Autodesk Inventor part; units mm, degrees
ref_plane "YZ Plane" through (0, 0, 0) normal (1, 0, 0) x (0, 1, 0)
ref_plane "XZ Plane" through (0, 0, 0) normal (0, 1, 0) x (-1, 0, 0)
ref_plane "XY Plane" through (0, 0, 0) normal (0, 0, 1) x (1, 0, 0)
sketch "Sketch1" plane through (0, 0, 0) normal (0, 1, 0) x (-1, 0, 0)
  circle A0 centre (0, 0) radius 12.3
  circle A1 centre (0, 0) radius 4.5
  circle A2 centre (0, 0) radius 2.75
  circle A3 centre (0, 0) radius 1.5
  dimension "d0" = 24.6
  dimension "d1" = 9
  dimension "d2" = 5.5
  dimension "d3" = 3
extrude "Extrusion1" add sketch "Sketch1" along normal blind 2 contours A0
sketch "Sketch2" plane through (0, 0, 0) normal (0, -1, 0) x (1, 0, 0)
  circle A0 centre (0, 0) radius 10
  circle A1 centre (0, 0) radius 4.5
  circle A2 centre (0, 0) radius 2.75
  circle A3 centre (0, 0) radius 1.5
  dimension "d6" = 20
  dimension "d7" = 9
  dimension "d8" = 5.5
  dimension "d9" = 3
extrude "Extrusion2" add sketch "Sketch2" against normal blind 4.5 contours A1
sketch "Sketch3" plane through (0, 0, 0) normal (0, -1, 0) x (1, 0, 0)
  circle A0 centre (0, 0) radius 10
  circle A1 centre (0, 0) radius 4.5
  circle A2 centre (0, 0) radius 2.75
  circle A3 centre (0, 0) radius 1.5
  dimension "d12" = 20
  dimension "d13" = 9
  dimension "d14" = 5.5
  dimension "d15" = 3
extrude "Extrusion3" add sketch "Sketch3" against normal blind 1 contours A2
sketch "Sketch4" plane through (0, 4.5, 0) normal (0, 1, 0) x (1, 0, 0)
  circle A0 centre (0, 0) radius 8.3 construction
  line L0 (0, 0) -> (0, -8.3) construction
  circle A1 centre (0, -8.3) radius 1.5
  dimension "d18" = 16.6
  dimension "d19" = 3
extrude "Extrusion4" cut sketch "Sketch4" against normal up to next
pattern_circular "Circular Pattern1" count 4 over 360 about axis through (0, 0, 0) along (0, 1, 0) of "Extrusion4"
sketch "Sketch5" plane through (0, 4.5, 0) normal (0, 1, 0) x (1, 0, 0)
  circle A0 centre (0, 0) radius 1.5
  circle A1 centre (0, 0) radius 3 construction
  line L0 (0, 0) -> (0, -3) construction
  line L1 (0, 0) -> (-0.376, -2.9763) construction
  line L2 (0, 0) -> (-0.7461, -2.9057) construction
  circle A2 centre (0, 0) radius 2.75
  line L3 (0, -2.75) -> (-0.376, -2.9763)
  line L4 (-0.6839, -2.6636) -> (-0.376, -2.9763)
  arc A3 (-0.6839, -2.6636) -> (0, -2.75) centre (0, 0) ccw
  dimension "d25" = 6
  dimension "d26" = 7.2
  dimension "d27" = 14.4
extrude "Extrusion5" cut sketch "Sketch5" against normal up to surface (3.5 mm away) contours A2 L3 L4
pattern_circular "Circular Pattern2" count 25 over 360 about axis through (0, 0, 0) along (0, 1, 0) of "Extrusion5"
properties part number "Horn"
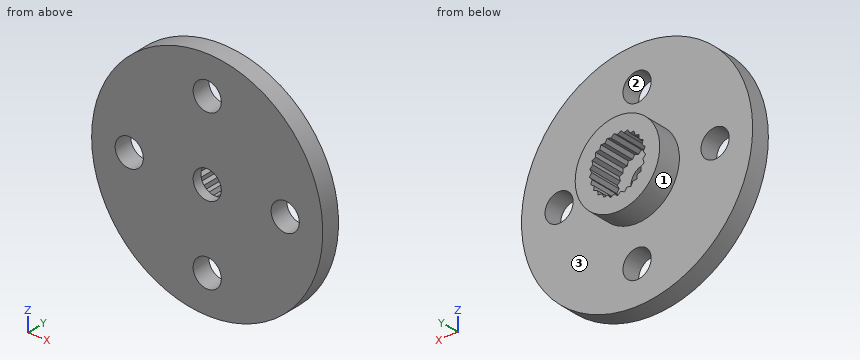
Work out the finished part from the listing and answer in its coordinate system (mm). Face numbers are marked on the shaded views. Coordinates: 2 decimals unless noted, no trailing zeros. Loops run counter-clockwise (first coordinate to the right, second up) from the corner with the lowest first, then second, coordinate; pieces in that order, holes last. Notation, with made-up numbers: (42, 29) -> (89, 29) arc R15 cw to (89, 55) -> close; hole circle Ø10 at (-33.75, 72). An arc over 180 degrees is marked (long way). Answer as CSV lines item,"result".
Q1. For a pull along X with two mould halves and no side action, classify the marked faces 1, 2 and 3 as +X half, -X half, draft (parallel to the pull), parting line (faces both ways), or undercut.
Findings:
face 1,"parting line"
face 2,"undercut"
face 3,"draft"
Q2. The part is cut by section A-A on z = 8.3. Write down the section's boundary in (x, y).
Findings:
outline,"(-9.08, 0) -> (-1.5, 0) -> (-1.5, 2) -> (-9.08, 2) -> close; (1.5, 0) -> (9.08, 0) -> (9.08, 2) -> (1.5, 2) -> close"
Q3. Find the intervals of material crossed by probe 1 along Z at (x, y) = (0, 0.6); probe 2 along Y at (x, z) = (-4, -6); probe 3 along Z at (x, y) = (-9, 1.5), in increasing order.
Findings:
probe 1,"z = -12.3 to -9.8, -6.8 to -1.5, 1.5 to 6.8, 9.8 to 12.3"
probe 2,"y = 0 to 2"
probe 3,"z = -8.38 to -1.33, 1.33 to 8.38"
Q4. The part is cut by section C-C on y = 1.55. State how many separate pieces and enclosed holes the cut face has, and give its area (3 significant figures).
Findings:
separate pieces,"1"
enclosed holes,"5"
area,"421 mm²"
Q5. The part is cut by section B-B on x = -8.3. Write down the section's boundary in (y, z).
Findings:
outline,"(0, -9.08) -> (2, -9.08) -> (2, -1.5) -> (0, -1.5) -> close; (0, 1.5) -> (2, 1.5) -> (2, 9.08) -> (0, 9.08) -> close"
Q6. Each of these flat-tipped pins is pushed along its axis until it touches: pin 1 (8 mm diameter, centred on x = -5, z = 1.5, fed in from +Y); pin 2 (4 mm diameter, centred on x = 0, z = 0, fed in from +Y); pin 3 (1 mm diameter, centred on x = -5, z = 4, fed in from +Y). Where does it stop, or does it pass through?
Findings:
pin 1,"stops at y = 4.5"
pin 2,"stops at y = 1"
pin 3,"stops at y = 2"
Q7. The part is cut by section D-D on x = -5.75. Write down the section's boundary in (y, z), and give its area (3 significant figures).
Findings:
outline,"(0, -10.87) -> (2, -10.87) -> (2, 10.87) -> (0, 10.87) -> close"
area,"43.5 mm²"
